```python
from build123d import *

# Parameters (mm, degrees)
SCHIZZO2_W                   = 10
SCHIZZO2_H                   = 35
ESTRUSIONE_ESTRUSIONE1_DEPTH = 71.3


with BuildPart() as part:
    # Schizzo1 → Rivoluzione1 (revolve)
    with BuildSketch(Plane.XY, mode=Mode.PRIVATE) as rivoluzione1_sk:
        Polygon((-152.5, 0), (152.5, 0), (152.5, 61.5), (87.5, 61.5), (87.5, 70), (80.5, 70), (80.5, 40), (35.5, 40), (35.5, 70), (26.8, 70), (26.8, 101), (-44.5, 101), (-44.5, 61.5), (-152.5, 61.5), align=None)
    revolve(rivoluzione1_sk.sketch.rotate(Axis((-1716.324322208, 0, 0), (1, 0, 0)), 90), axis=Axis((-1716.324322208, 0, 0), (1, 0, 0)))

    # Schizzo2 → Estrusione-Estrusione1 (add)
    with BuildSketch(Plane.ZY.offset(44.5)):
        with Locations((0, 95)):
            Rectangle(SCHIZZO2_W, SCHIZZO2_H)
    extrude(amount=-ESTRUSIONE_ESTRUSIONE1_DEPTH)


solid = part.part
```
The listing builds one solid part. Answer for the finished solid, in the listing's coordinates (mm). A direction names the side the tool comes from. Give positions to 0.01 mm unless a question says otherwise; leave off trailing zeros. Write each loop counter-clockwise with the first axis right and the second up, starting at its lowest first coordinate (ties: lowest second). Pieces come first, ordered by that corner, then holes. Notation, with made-up numbers: M -23,9.5 L 29,9.5 A20 ccw 29,31.5 Z; hole C 73,44.25 d2. An arc over 180 degrees is marked long. Write each question's results on one line, items separated by ' | '.
Q1. Section B-B, the plane z = 0 is taken. Write down the section's boundary in (x, y), then the cut area to 3 significant figures.
Output values:
outline: M -152.5,-61.5 L -44.5,-61.5 L -44.5,-101 L 26.8,-101 L 26.8,-70 L 35.5,-70 L 35.5,-40 L 80.5,-40 L 80.5,-70 L 87.5,-70 L 87.5,-61.5 L 152.5,-61.5 L 152.5,61.5 L 87.5,61.5 L 87.5,70 L 80.5,70 L 80.5,40 L 35.5,40 L 35.5,70 L 26.8,70 L 26.8,112.5 L -44.5,112.5 L -44.5,61.5 L -152.5,61.5 Z | area: 42,300 mm2
Q2. A tool of negligible diameter and unlimited length cuts with its end or side. For faces 1 (the cylindrical face through (57.68, -1.76, -39.96)), 2 (the flat face through (-9, 107, -5)), 3 (the cylindrical face through (119.545, -60.977, -8.006)), from which of +Z, -Z, +X, -X, +Y, -Y can it reach the whole face along a straight path? Write none if from no direction.
Output values:
face 1: none | face 2: -Z, +X, -X, +Y | face 3: +X
Q3. Flat-ended cylindrical pins translate along their axes: P1, Ø3, axis at x = -63.5, y = 34, coming from the +Z side; P2, Ø8, axis at y = 45.5, z = -60.5, coming from the -X side; P3, Ø5, axis at x = 9, y = -63, coming from the +Z side. Find the tip coordinate at first contact, or state that the pin passes through.
Output values:
P1: z = 52.21 | P2: x = -44.5 | P3: z = 80.87
Q4. Consider L1, parallel to X at y = -56, z = 5; L2, parallel to X at y = -25, z = -63; L3, parallel to X at y = 19.5, z = -81. Determine where each line is inside the solid, lowest interval first. Write a range as from..to.
Output values:
L1: -152.5..35.5, 80.5..152.5 | L2: -44.5..35.5, 80.5..87.5 | L3: -44.5..26.8
Q5. Section D-D, the plane x = 95.5 is taken. Write down the section's boundary in (y, z), then the cut area to 3 significant figures.
Output values:
outline: C 0,0 d123 | area: 11,900 mm2
Q6. Section A-A, the plane y = -56 is taken. Write down the section's boundary in (x, z).
Output values:
outline: M -152.5,-25.42 L -44.5,-25.42 L -44.5,-84.05 L 26.8,-84.05 L 26.8,-42 L 35.5,-42 L 35.5,42 L 26.8,42 L 26.8,84.05 L -44.5,84.05 L -44.5,25.42 L -152.5,25.42 Z; M 80.5,-42 L 87.5,-42 L 87.5,-25.42 L 152.5,-25.42 L 152.5,25.42 L 87.5,25.42 L 87.5,42 L 80.5,42 Z
Q7. Section C-C, the plane z = 50 is taken. Write down the section's boundary in (x, y), then the cut area to 3 significant figures.
Output values:
outline: M -152.5,-35.81 L -44.5,-35.81 L -44.5,-87.76 L 26.8,-87.76 L 26.8,-48.99 L 35.5,-48.99 L 35.5,48.99 L 26.8,48.99 L 26.8,87.76 L -44.5,87.76 L -44.5,35.81 L -152.5,35.81 Z; M 80.5,-48.99 L 87.5,-48.99 L 87.5,-35.81 L 152.5,-35.81 L 152.5,35.81 L 87.5,35.81 L 87.5,48.99 L 80.5,48.99 Z | area: 26,400 mm2
